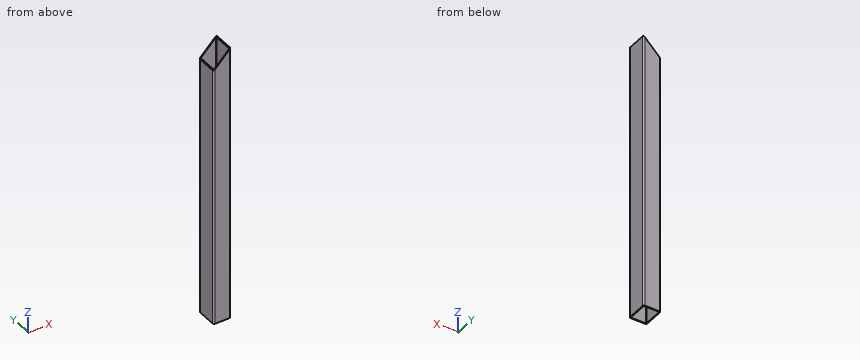
Autodesk Inventor part; units mm, degrees
ref_plane "Start plane" through (0, 0, 0) normal (0, 0, 1) x (1, 0, 0)
ref_plane "End plane" through (0, 0, 650) normal (0, 0, 1) x (1, 0, 0)
ref_plane "Work Plane5" through (20, 0, 650) normal (-0.7071, 0, 0.7071) x (0.7071, 0, 0.7071)
ref_plane "Start plane" through (0, 0, 0) normal (0, 0, 1) x (1, 0, 0)
ref_plane "End plane" through (0, 0, 650) normal (0, 0, 1) x (1, 0, 0)
sketch "Sketch" plane through (0, 0, 0) normal (0, 0, 1) x (1, 0, 0)
  line L0 (-20, -22) -> (-20, 22)
  line L1 (-17, 25) -> (17, 25)
  line L2 (20, 22) -> (20, -22)
  line L3 (17, -25) -> (-17, -25)
  arc A0 (-20, -22) -> (-17, -25) centre (-17, -22) ccw
  arc A1 (-17, 25) -> (-20, 22) centre (-17, 22) ccw
  arc A2 (20, 22) -> (17, 25) centre (17, 22) ccw
  arc A3 (17, -25) -> (20, -22) centre (17, -22) ccw
  arc A4 (-17, 23) -> (-18, 22) centre (-17, 22) ccw
  line L4 (-17, 23) -> (17, 23)
  arc A5 (18, 22) -> (17, 23) centre (17, 22) ccw
  line L5 (18, 22) -> (18, -22)
  arc A6 (17, -23) -> (18, -22) centre (17, -22) ccw
  line L6 (17, -23) -> (-17, -23)
  arc A7 (-18, -22) -> (-17, -23) centre (-17, -22) ccw
  line L7 (-18, -22) -> (-18, 22)
  line L8 (0, 35.8698) -> (0, -35.8698) construction
  line L9 (-28.8698, 0) -> (28.8698, 0) construction
  dimension "d7" = 3
  dimension "d10" = 50
  dimension "d11" = 40
  dimension "d12" = 2
  dimension "d15" = 25
  dimension "d16" = 20
extrude "Body" add sketch "Sketch" along normal up to surface (650 mm away) from surface at 0
sketch "Sketch3" plane through (0, 0, 0) normal (0, 0, 1) x (1, 0, 0)
  line L0 (0, 0) -> (10, 0)
ref_plane "Work Plane3" through (0, 0, 0) normal (0, -1, 0) x (1, 0, 0)
sketch "Sketch4" plane through (0, 0, 0) normal (0, -1, 0) x (1, 0, 0)
  line L0 (-2, 0) -> (12, 0)
  line L1 (-2, 650) -> (12, 650)
  dimension "d18" = 650
ref_plane "Work Plane5" through (20, 0, 650) normal (-0.7071, 0, 0.7071) x (0.7071, 0, 0.7071)
split "Split2" plane through (20, 0, 650) removes the side toward (-0.7071, 0, 0.7071)
equation "\"d7\" = G_IR"
equation "\"d10\" = G_H"
equation "\"d11\" = G_W"
equation "\"d12\" = G_T"
equation "\"d15\" = 0.5 * d10"
equation "\"d16\" = 0.5 * d11"
equation "\"d3\" = G_L"
equation "\"G_W\" = 40"
equation "\"G_H\" = 50"
equation "\"G_T\" = 2"
equation "\"G_IR\" = 3"
equation "\"G_L\" = d18"
equation "\"G_OFFSET_START\" = 0"
equation "\"G_OFFSET_END\" = 0"
equation "\"d14\" = G_OFFSET_END + B_L"
equation "\"B_L\" = 650"
properties part number "UNI EN 10305-5 - 50 x 40 x 2  - 650" material "Steel, Mild"
Could you check a few things on this model? Use its own coordinates, in mm. Coordinates: 2 decimals unless noted, no trailing zeros. Write each loop counter-clockwise with the first axis right and the second up, starting at its lowest first coordinate (ties: lowest second). Pieces come first, ordered by that corner, then holes. Notation, with made-up numbers: (37.5, -12) -> (71.5, -12) arc R19 ccw to (71.5, 6) -> close; hole circle Ø7 at (-39, 20.25). An arc over 180 degrees is marked (long way). Write item = value, one per line. Start each with the question number.
(1) I want a section at B-B (z = 179). Please give me the cut outline in (x, y).
(2) I want a section at A-A (x = 9.5). Please give me the cut outline in (y, z).
(3) I need wall thicknesses on line 1 (X direction, y = -15, z = 463.5); line 2 (Y direction, x = -11, z = 340); line 3 (X direction, y = 22.5, z = 496). Which ranges of each line are inside material? Lowest first, please. Write a range as [from, to].
(4) I want a section at C-C (y = 16). Please give me the cut outline in (x, z).
Result set:
q1.outline = (-20, -22) arc R3 ccw to (-17, -25) -> (17, -25) arc R3 ccw to (20, -22) -> (20, 22) arc R3 ccw to (17, 25) -> (-17, 25) arc R3 ccw to (-20, 22) -> close; hole (-18, -22) arc R1 ccw to (-17, -23) -> (17, -23) arc R1 ccw to (18, -22) -> (18, 22) arc R1 ccw to (17, 23) -> (-17, 23) arc R1 ccw to (-18, 22) -> close
q2.outline = (-25, 0) -> (-23, 0) -> (-23, 639.5) -> (-25, 639.5) -> close; (23, 0) -> (25, 0) -> (25, 639.5) -> (23, 639.5) -> close
q3.line_1 = [-20, -18], [18, 20]
q3.line_2 = [-25, -23], [23, 25]
q3.line_3 = [-19.96, -17.87], [17.87, 19.96]
q4.outline = (-20, 0) -> (-18, 0) -> (-18, 612) -> (-20, 610) -> close; (18, 0) -> (20, 0) -> (20, 650) -> (18, 648) -> close
